Could you check a few things on this model? Use its own coordinates, in mm. A direction names the side the tool comes from. Coordinates: 2 decimals unless noted, no trailing zeros. Write each loop counter-clockwise with the first axis right and the second up, starting at its lowest first coordinate (ties: lowest second). Pieces come first, ordered by that corner, then holes.
```python
from build123d import *

# Parameters (mm, degrees)
SKETCH_1_R          = 10
SKETCH_1_R_2        = 3
SKETCH_1_R_3        = 1.6
SKETCH_1_R_4        = 1.600000000000001
SKETCH_1_R_5        = 1.6000000000000003
SKETCH_1_R_6        = 1.6000000000000019
EXTRUDE_1_DEPTH     = 3
EXTRUDE_2_DEPTH     = 3
SKETCH_3_R          = 1.5999999999999974
EXTRUDE_3_DEPTH     = 3
FILLET_1_R          = 10
FILLET_2_R          = 20
CUT_EXTRUDE_START   = -3
SKETCH_4_R          = 1.6000000000000019
SKETCH_4_R_2        = 1.599999999999998
CUT_EXTRUDE_1_DEPTH = 3
FILLET_3_R          = 5
FILLET_4_R          = 2


with BuildPart() as part:
    # 草图1 → 凸台-拉伸1 (new body)
    with BuildSketch(Plane(origin=(0, 0, 0), x_dir=(1, 0, 0), z_dir=(0, 1, 0))):
        with Locations(Location((0, 0, 0), (0, 0, 270))):
            Circle(SKETCH_1_R)
        with Locations(Location((0, 0, 0), (0, 0, 270))):
            Circle(SKETCH_1_R_2, mode=Mode.SUBTRACT)
        with Locations(Location((0, 6.999999999999999, 0), (0, 0, 270))):
            Circle(SKETCH_1_R_3, mode=Mode.SUBTRACT)
        with Locations(Location((6.999999999999998, 0, 0), (0, 0, 270))):
            Circle(SKETCH_1_R_4, mode=Mode.SUBTRACT)
        with Locations(Location((8.7e-16, -6.999999999999999, 0), (0, 0, 270))):
            Circle(SKETCH_1_R_5, mode=Mode.SUBTRACT)
        with Locations(Location((-6.999999999999999, -8.7e-16, 0), (0, 0, 270))):
            Circle(SKETCH_1_R_6, mode=Mode.SUBTRACT)
    extrude(amount=EXTRUDE_1_DEPTH)

    # 草图2 → 凸台-拉伸2 (add)
    with BuildSketch(Plane(origin=(0, 3, 0), x_dir=(1, 0, 0), z_dir=(0, 1, 0))):
        Polygon((-8.000000000000005, -5.999999999999994), (-57.4, -6), (-57.4, 6), (-8.000000000000005, 5.999999999999994), align=None)
    extrude(amount=-EXTRUDE_2_DEPTH)

    # 草图3 → 凸台-拉伸3 (add)
    with BuildSketch(Plane(origin=(0, 3, 0), x_dir=(1, 0, 0), z_dir=(0, 1, 0))):
        Polygon((-57.4, -6), (-37.399999999999984, -6), (-37.39999999999999, -40), (-57.39999999999999, -40), align=None)
        with Locations(Location((-52.89999999999999, -34.5, 0), (0, 0, 270))):
            Circle(SKETCH_3_R, mode=Mode.SUBTRACT)
        with Locations(Location((-41.89999999999999, -34.5, 0), (0, 0, 270))):
            Circle(SKETCH_3_R, mode=Mode.SUBTRACT)
    extrude(amount=-EXTRUDE_3_DEPTH)

    # 圆角1
    fillet_1_edges = [part.edges().sort_by_distance(p)[0] for p in [
        (-37.399999999999984, 1.5, 6),
    ]]
    fillet(fillet_1_edges, radius=FILLET_1_R)

    # 圆角2
    fillet_2_edges = [part.edges().sort_by_distance(p)[0] for p in [
        (-57.4, 1.5, -6),
    ]]
    fillet(fillet_2_edges, radius=FILLET_2_R)

    # 草图4 → 切除-拉伸1 (cut)
    with BuildSketch(Plane(origin=(0, 3, 0), x_dir=(1, 0, 0), z_dir=(0, 1, 0)).offset(CUT_EXTRUDE_START)):
        with Locations(Location((-6.999999999999999, -8.7e-16, 0), (0, 0, 270))):
            Circle(SKETCH_4_R)
        with Locations(Location((-32, 0, 0), (0, 0, 270))):
            Circle(SKETCH_4_R_2)
        with BuildLine():
            Line((-24.999999999999996, 3), (-13.999999999999998, 3))
            ThreePointArc((-13.999999999999998, 3), (-10.999999999999998, 0), (-13.999999999999998, -3))
            Line((-13.999999999999998, -3), (-24.999999999999996, -3))
            ThreePointArc((-24.999999999999996, -3), (-27.999999999999996, 3.7e-16), (-24.999999999999996, 3))
        make_face()
        with BuildLine():
            Line((-51.399999999999984, -23.500000000000004), (-43.39999999999999, -23.500000000000004))
            ThreePointArc((-43.39999999999999, -23.500000000000004), (-39.89999999999999, -27.000000000000004), (-43.39999999999999, -30.500000000000004))
            Line((-43.39999999999999, -30.500000000000004), (-51.399999999999984, -30.500000000000004))
            ThreePointArc((-51.399999999999984, -30.500000000000004), (-54.899999999999984, -27.000000000000004), (-51.399999999999984, -23.500000000000004))
        make_face()
        with BuildLine():
            Line((-40.43840481040531, -12.5), (-40.43840481040531, -17.500000000000004))
            Line((-40.43840481040531, -17.500000000000004), (-53.93871883229112, -17.500000000000007))
            Line((-53.93871883229112, -17.500000000000007), (-53.938718832291116, -12.5))
            ThreePointArc((-53.938718832291116, -12.5), (-48.18321723568186, -1.3706117859306186), (-36.28930043689978, 2.5694166190035115))
            ThreePointArc((-36.28930043689978, 2.5694166190035115), (-36.81589304125609, -1.3443117998370948), (-34.338414417674585, -4.419481645081424))
            ThreePointArc((-34.338414417674585, -4.419481645081424), (-38.17460072758567, -7.866244461436596), (-40.43840481040531, -12.5))
        make_face()
    extrude(amount=CUT_EXTRUDE_1_DEPTH, mode=Mode.SUBTRACT)

    # 圆角3
    fillet_3_edges = [part.edges().sort_by_distance(p)[0] for p in [
        (-8.000000000000005, 1.5, -5.999999999999994),
        (-8.000000000000005, 1.5, 5.999999999999994),
        (-57.39999999999999, 1.5, 40),
        (-37.39999999999999, 1.5, 40),
    ]]
    fillet(fillet_3_edges, radius=FILLET_3_R)

    # 圆角4
    # the kernel refuses this fillet: 2 mm, written as the material it adds along each edge
    with BuildSketch(Plane(origin=(-36.28930043689978, 0, -2.5694166190035155), x_dir=(-0.9997848253310014, 0, 0.020743746958035388), z_dir=(0, 1, 0))) as fillet_4_piece_1:
        with BuildLine():
            CenterArc((2.7332128689398965, 1.9923174543114084), FILLET_4_R, 174.54438439769004, 100.47920721380297)
            ThreePointArc((0.7422725749788821, 2.1824667269433027), (0.49863093433961686, 1.0478715203584514), (0, 0))
            ThreePointArc((0, 0), (1.4541723542762737, -0.06379048821461454), (2.9083447085525433, 0))
        make_face()
    extrude(amount=3)
    with BuildSketch(Plane(origin=(-34.338414417674585, 0, 4.419481645081424), x_dir=(-0.7648370504250814, 0, -0.6442237858827173), z_dir=(0, 1, 0))) as fillet_4_piece_2:
        with BuildLine():
            CenterArc((2.5407101067548044, 1.9546581979795647), FILLET_4_R, 170.9703370053984, 86.80615278737906)
            ThreePointArc((0.5654956678276036, 2.2685497720198655), (0.33194950705873716, 1.1220100755321154), (0, 0))
            ThreePointArc((0, 0), (1.0586292111478346, 0.11335450505108799), (2.117258422295671, -7e-17))
        make_face()
    extrude(amount=3)
    with BuildSketch(Plane(origin=(-40.43840481040531, 0, 17.500000000000004), x_dir=(0, 0, -1), z_dir=(0, 1, 0))) as fillet_4_piece_3:
        with BuildLine():
            CenterArc((FILLET_4_R, FILLET_4_R), FILLET_4_R, 180, 90)
            Line((0, FILLET_4_R), (0, 0))
            Line((0, 0), (FILLET_4_R, 0))
        make_face()
    extrude(amount=3)
    with BuildSketch(Plane(origin=(-53.93871883229112, 0, 17.500000000000007), x_dir=(1, 0, 0), z_dir=(0, 1, 0))) as fillet_4_piece_4:
        with BuildLine():
            CenterArc((FILLET_4_R, FILLET_4_R), FILLET_4_R, 179.99999999999986, 90.00000000000011)
            Line((7.11e-15, FILLET_4_R), (0, 0))
            Line((0, 0), (FILLET_4_R, 0))
        make_face()
    extrude(amount=3)
    with BuildSketch(Plane(origin=(-53.938718832291116, 0, 12.5), x_dir=(0.09331197212510238, 0, -0.9956369196941844), z_dir=(0, 1, 0))) as fillet_4_piece_5:
        with BuildLine():
            CenterArc((0.09361195431707342, -1.9999910052952001), FILLET_4_R, 89.8281631699166, 5.526008171417317)
            Line((-0.09301198993312956, -0.00871716590683111), (0, 0))
            ThreePointArc((0, 0), (0.04980509112364704, 7.468574010459e-05), (0.09961018224729987, 0))
        make_face()
    extrude(amount=3)
    # the kernel refuses this fillet: 2 mm, written as the material it takes off along each edge
    with BuildSketch(Plane(origin=(-40.43840481040531, -0.7436301227400532, 12.500000000000004), x_dir=(0.26988358130767626, 0, -0.9628929600638604), z_dir=(0, 1, 0))) as fillet_4_2_piece_1:
        with BuildLine():
            CenterArc((0.2754185639777855, -1.9998786277005756), FILLET_4_R, 89.36877437844454, 16.28856500222963)
            Line((-0.2643485986375687, -0.0740927075728552), (0, 0))
            ThreePointArc((0, 0), (0.14872602454800565, 0.00081926302110449), (0.29745204909602135, 1e-17))
        make_face()
    extrude(amount=4.4872602454801065, mode=Mode.SUBTRACT)


solid = part.part
```
1. On a 3-axis mill with a long thin cutter (end or side, diameter ignored), from which of +Z, -Z, +X, -X, +Y, -Y can I reach the whole of each face in a straight line? I mean faces 4 (the face through (-34.55, 1.48, 9.01)), 5 (the face through (-37.4, 2, 25)), 6 (the face through (-47, 1, 23.5)). Say none if no direction works.
Verdict:
face 4: +Z, +Y, -Y
face 5: +Z, +X, +Y, -Y
face 6: +Y, -Y
2. For pin 1 (1 mm diameter, centred on y = 2.5, z = 5.5, fed in from -X); pin 2 (1 mm diameter, centred on y = 1.5, z = 16.5, fed in from +X); pin 3 (0.9 mm diameter, centred on x = -49.5, y = 2, fed in from -Z), each with a flat end and sliding along its axis, tell me the tip position at first contact or that it passes through.
Verdict:
pin 1: stops at x = -55.73
pin 2: stops at x = -37.4
pin 3: stops at z = -2.26
3. Please list where these lines run through material, in increasing order: line 1 along X through (y, z) = (1.3, 34.5); line 2 along Z through (x, y) = (-22, 2.7); line 3 along X through (y, z) = (1.1, 34).
Verdict:
line 1: x = -57.4 to -54.5, -51.3 to -43.5, -40.3 to -37.4
line 2: z = -6 to -3, 3 to 6
line 3: x = -57.4 to -54.42, -51.38 to -43.42, -40.38 to -37.4
4. I want a section at A-A on x = 0. Please give me the cut outline in (y, z), plus the area to 3 significant figures.
Verdict:
outline: (0, -10) - (3, -10) - (3, -8.6) - (0, -8.6) - close; (0, -5.4) - (3, -5.4) - (3, -3) - (0, -3) - close; (0, 3) - (3, 3) - (3, 5.4) - (0, 5.4) - close; (0, 8.6) - (3, 8.6) - (3, 10) - (0, 10) - close
area: 22.8 mm2
5. I want a section at B-B on x = 7. Please give me the cut outline in (y, z).
Verdict:
outline: (0, -7.14) - (3, -7.14) - (3, -1.6) - (0, -1.6) - close; (0, 1.6) - (3, 1.6) - (3, 7.14) - (0, 7.14) - close
6. I want a section at C-C on z = 31.5. Please give me the cut outline in (x, y), plus the area to 3 significant figures.
Verdict:
outline: (-57.4, 0) - (-37.4, 0) - (-37.4, 3) - (-57.4, 3) - close
area: 60.0 mm2
7. I want a section at D-D on y = 1.7. Give the number of separate pieces and of enclosed holes in the cut face, plus the area to 3 significant figures.
Verdict:
separate pieces: 1
enclosed holes: 11
area: 968 mm2
8. If we mould it in two halves opening along X, with no side actions, what happens to faces 1 (the face through (-53.368, 1.479, 16.899)), 2 (the face through (-34, 0, 8)), 3 (the face through (-55.97, 1.48, 38.5))? For each: pulls with the +X half, pulls with the -X half, needs draft (parallel to the pull), parting line crosses it, or undercut.
Verdict:
face 1: undercut
face 2: needs draft
face 3: pulls with the -X half
